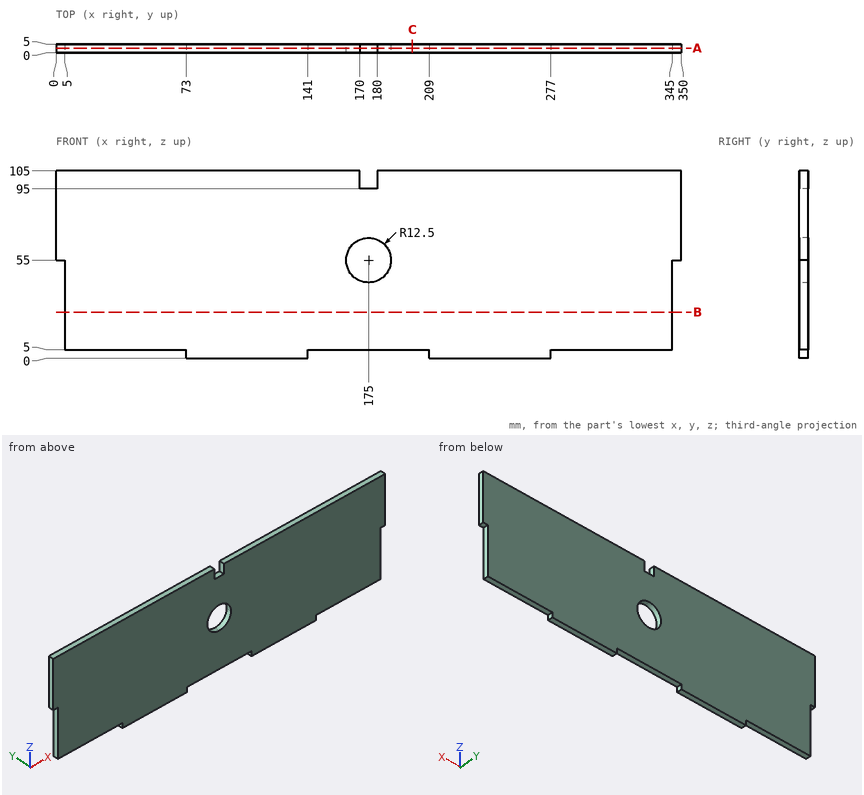
Could you check a few things on this drawing? It's one solid part, dimensions in mm from its lowest x, y, z. Round coordinates to 2 decimals unless told otherwise and drop trailing zeros. Order: outer loops, then holes, each group sorted by start corner. A loop starts at its lowest first (then second) coordinate and runs counter-clockwise, first axis right, second up. Notation, with made-up numbers: M -26.75,-15.75 L 14.25,-15.75 A14 cw 14.25,-1.75 Z; hole C -28.75,74 d6. An arc over 180 degrees is marked long. One line per item, written item: value.
(1) I need wall thicknesses on line 1 along Z through (x, y) = (176, 1.85); line 2 along Z through (x, y) = (19, 3); line 3 along X through (y, z) = (3.95, 26). Which ranges of each line are inside material? Lowest first, please. Write a range as from..to.
Ans:
line 1: z = 5..42.54, 67.46..95
line 2: z = 5..105
line 3: x = 5..345
(2) Imagine slicing it at C-C (x = 199.5). Write out the boundary of the cut face in (y, z), and give its area (3 significant figures).
Ans:
outline: M 0,5 L 5,5 L 5,105 L 0,105 Z
area: 500 mm^2
(3) I'm going to push flat-ended pins straight in: P1, Ø2.5, axis at x = 191, y = 3.5, coming from the -Z side; P2, Ø2, axis at x = 202, z = 64.5, coming from the -Y side; P3, Ø1.5, axis at y = 4.5, z = 49, coming from the +X side; P4, Ø2.5, axis at y = 2.5, z = 1.5, coming from the +X side. Where does each tip first touch, or does it pass through?
Ans:
P1: stops at z = 5
P2: stops at y = 0
P3: stops at x = 345
P4: stops at x = 277
(4) Imagine slicing it at A-A (y = 2.7). Write out the boundary of the cut face in (x, z), and give its area (3 significant figures).
Ans:
outline: M 0,55 L 5,55 L 5,5 L 73,5 L 73,0 L 141,0 L 141,5 L 209,5 L 209,0 L 277,0 L 277,5 L 345,5 L 345,55 L 350,55 L 350,105 L 180,105 L 180,95 L 170,95 L 170,105 L 0,105 Z; hole M 175,42.5 A12.5 ccw 187.5,55 A12.5 ccw long Z
area: 34,600 mm^2
(5) Imagine slicing it at B-B (z = 26). Write out the boundary of the cut face in (x, y).
Ans:
outline: M 5,0 L 345,0 L 345,5 L 5,5 Z
